```python
from build123d import *

# Parameters (mm, degrees)
CROQUIS1_R              = 3.99
SALIENTE_EXTRUIR1_DEPTH = 50
CROQUIS2_W              = 1
CROQUIS2_H              = 0.8
CHAFL_N1_SIZE           = 0.5


with BuildPart() as part:
    # Croquis1 → Saliente-Extruir1 (new body)
    with BuildSketch(Plane.XY):
        Circle(CROQUIS1_R)
    extrude(amount=SALIENTE_EXTRUIR1_DEPTH)

    # Croquis2 → Cortar-Revolución1 (revolve, cut)
    with BuildSketch(Plane(origin=(0, 0, 0), x_dir=(0, 0, -1), z_dir=(1, 0, 0))):
        with Locations((-15.2, 3.59)):
            Rectangle(CROQUIS2_W, CROQUIS2_H)
        with Locations((-32.2, 3.59)):
            Rectangle(CROQUIS2_W, CROQUIS2_H)
    revolve(axis=Axis((0, 0, 50), (0, 0, -1)), mode=Mode.SUBTRACT)

    # Chaflán1
    chafl_n1_edges = [part.edges().sort_by_distance(p)[0] for p in [
        (-3.99, 0, 0),
        (-3.99, 0, 50),
    ]]
    chamfer(chafl_n1_edges, length=CHAFL_N1_SIZE)


solid = part.part
```
Verification items for the finished model (mm, model axes). A direction names the side the tool comes from. Round coordinates to 2 decimals unless told otherwise and drop trailing zeros. Order: outer loops, then holes, each group sorted by start corner. A loop starts at its lowest first (then second) coordinate and runs counter-clockwise, first axis right, second up. Notation, with made-up numbers: (-32, 79) -> (20, 79) arc R25 cw to (20, 103) -> close; hole circle Ø8 at (49.25, 61.5). An arc over 180 degrees is marked (long way). Put each result on its own line as item: value. Start each with the question number.
(1) Material ranges on line 1 along Z through (x, y) = (3.25, -1.25); line 2 along Z through (x, y) = (-3, 2.5); line 3 along Y through (x, z) = (-0.25, 47), recorded low to high.
(2) Draft check along Z on faces 3 (the face through (3.806, 1.198, 7.501)), 4 (the face through (0, 0, 0)), 5 (the face through (0, 0, 50)), 6 (the face through (-2, 3, 14.7)). Enter one of: +Z half, -Z half, draft (parallel to the pull), parting line (faces both ways), or undercut.
(3) Section check A-A (z = 22.5). Enter the section's corners in (x, y), then the cut area to 3 significant figures.
(4) Tool access check on faces 1 (the face through (0.958, 3.043, 15.193)), 2 (the face through (3.806, 1.198, 23.588)). Record the directions out of +Z, -Z, +X, -X, +Y, -Y that give a thin tool (end or side, any length) a straight path to the whole face; none if there is none.
(5) Depth check by flat-ended pin: pin 1 Ø1.5 at (x, z) = (-2.5, 7) entering from +Y. Enter the tip coordinate at first touch or a pass-through.
Completed:
1. line 1: z = 0 to 14.7, 15.7 to 31.7, 32.7 to 50
1. line 2: z = 0.42 to 14.7, 15.7 to 31.7, 32.7 to 49.58
1. line 3: y = -3.98 to 3.98
2. face 3: draft
2. face 4: -Z half
2. face 5: +Z half
2. face 6: undercut
3. outline: circle Ø7.98 at (0, 0)
3. area: 50.0 mm2
4. face 1: none
4. face 2: +Z, -Z
5. pin 1: stops at y = 3.59
